Drawing for the job (mm, zero at the part's lowest x, y, z). Coordinates: 2 decimals unless noted, no trailing zeros. Loops run counter-clockwise (first coordinate to the right, second up) from the corner with the lowest first, then second, coordinate; pieces in that order, holes last. Notation, with made-up numbers: (4.5, -31) - (29.5, -31) arc R24 cw to (29.5, 4) - close; hole circle Ø7 at (56, -21.5). An arc over 180 degrees is marked (long way). Put each result on its own line as item: value.
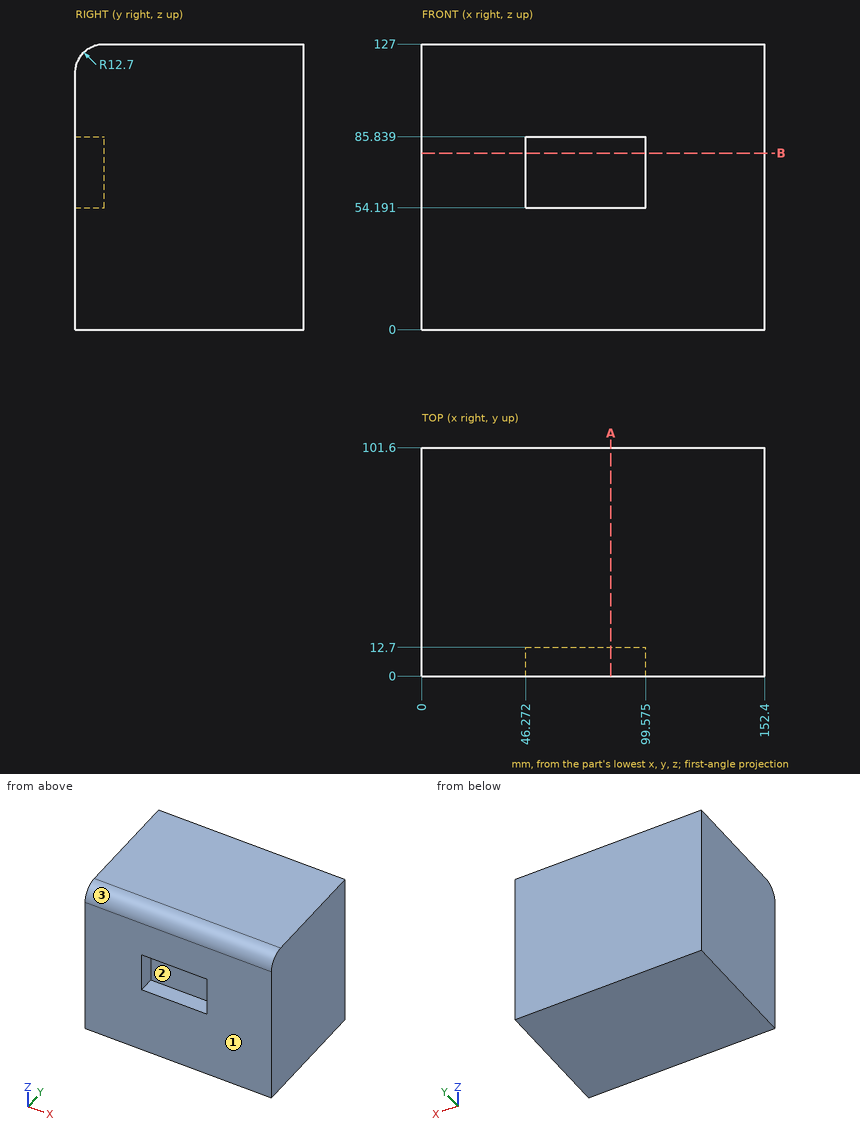
Q1. Wall check: L1, parallel to Y at x = 72.5, z = 72.5; L2, parallel to Z at x = 55, y = 9; L3, parallel to Y at x = 72.5, z = 117. Give the ranges that are in metal, low to high. Write a range as from..to.
Determined:
L1: 12.7..101.6
L2: 0..54.19, 85.84..126.45
L3: 0.29..101.6
Q2. Slice it at A-A, the plane x = 84. Give the cut face in (y, z), then the cut area to 3 significant figures.
Determined:
outline: (0, 0) - (101.6, 0) - (101.6, 127) - (12.7, 127) arc R12.7 ccw to (0, 114.3) - (0, 85.84) - (12.7, 85.84) - (12.7, 54.19) - (0, 54.19) - close
area: 12,500 mm2
Q3. Pin check, flat tips, straight feed: pin 1 Ø9.5 at (x, z) = (63.5, 63) entering from -Y; pin 2 Ø4 at (x, y) = (72.5, 5.5) entering from +Z. Stop position of each tip, or through.
Determined:
pin 1: y = 12.7
pin 2: z = 125.89
Q4. Slice it at B-B, the plane z = 78.5. Give the cut face in (x, y) (1 decimal).
Determined:
outline: (0, 0) - (46.3, 0) - (46.3, 12.7) - (99.6, 12.7) - (99.6, 0) - (152.4, 0) - (152.4, 101.6) - (0, 101.6) - close
Q5. Mould opens along Z. For the marked faces 1, 2 and 3 say: +Z half, -Z half, draft (parallel to the pull), parting line (faces both ways), or undercut.
Determined:
face 1: draft
face 2: undercut
face 3: +Z half
